Autodesk Inventor part; units mm, degrees
ref_plane "YZ Plane" through (0, 0, 0) normal (1, 0, 0) x (0, 1, 0)
ref_plane "XZ Plane" through (0, 0, 0) normal (0, 1, 0) x (-1, 0, 0)
ref_plane "XY Plane" through (0, 0, 0) normal (0, 0, 1) x (1, 0, 0)
sketch "Sketch1" plane through (0, 0, 0) normal (0, 1, 0) x (-1, 0, 0)
  circle A0 centre (0, 0) radius 45 construction
  line L0 (36.9, 6.3) -> (13, 6.3)
  line L1 (13, 6.3) -> (13, -6.3)
  line L2 (13, -6.3) -> (36.9, -6.3)
  line L3 (36.9, -6.3) -> (36.9, 6.3)
  line L4 (-12.994, 35.1063) -> (-23.906, 28.8063)
  line L5 (-23.906, 28.8063) -> (-11.956, 8.1083)
  line L6 (-1.044, 14.4083) -> (-12.994, 35.1063)
  line L7 (-11.956, 8.1083) -> (-1.044, 14.4083)
  line L8 (-18.9106, -20.1539) -> (-7.9987, -26.4539)
  line L9 (-7.9987, -26.4539) -> (3.9513, -5.7559)
  line L10 (-6.9606, 0.5441) -> (-18.9106, -20.1539)
  line L11 (3.9513, -5.7559) -> (-6.9606, 0.5441)
  circle A1 centre (11.0177, 0) radius 18 construction
  circle A2 centre (-5.5088, 9.5416) radius 18 construction
  circle A3 centre (-5.5088, -9.5416) radius 18 construction
  circle A4 centre (17, -29.4449) radius 1.8
  line L12 (0, 0) -> (20.2687, -35.1063)
  circle A5 centre (17, 29.4449) radius 1.8
  circle A6 centre (-34, 0) radius 1.8
  circle A7 centre (0, 0) radius 49
  line L13 (-5.5088, -9.5416) -> (-0.5088, -0.8813) construction
  line L14 (-5.5088, -9.5416) -> (4.4912, -9.5416) construction
  line L15 (-18.45, -31.9563) -> (3.4912, 6.0469) construction
  line L16 (-17.931, -18.4573) -> (-7.019, -24.7573) construction
  point P0 (-12.475, -21.6073)
  point P1 (-7.4794, -12.9547)
  dimension "d0" = 90
  dimension "d1" = 12.6
  dimension "d2" = 23.9
  dimension "d3" = 13
  dimension "d4" = 38.7
  dimension "d7" = 360
  dimension "d9" = 36
  dimension "d12" = 360
  dimension "d14" = 3.6
  dimension "d15" = 34
  dimension "d16" = -0.544
  dimension "d19" = 360
  dimension "d21" = 98
  dimension "d38" = 10
  dimension "d39" = 60
  dimension "d40" = 14.9588
extrude "Extrusion1" add sketch "Sketch1" along normal blind 7
sketch "Sketch2" plane through (0, 7, 0) normal (0, 1, 0) x (1, 0, 0)
  circle A0 centre (0, 0) radius 39.9 construction
  line L0 (1.044, -14.4083) -> (11.956, -8.1083) construction
  line L1 (6.5, -11.2583) -> (23.7787, -41.1859) construction
  circle A1 centre (19.95, -34.5544) radius 0.8
  circle A2 centre (14.95, 25.8942) radius 0.8
  circle A3 centre (-39.9, 0) radius 0.8
  line L2 (12.994, -35.1063) -> (1.044, -14.4083) construction
  line L3 (7.019, -24.7573) -> (17.931, -18.4573) construction
  line L4 (11.956, -8.1083) -> (23.906, -28.8063) construction
  circle A4 centre (5, -8.6603) radius 0.8
  circle A5 centre (0, 0) radius 0.8
  circle A6 centre (-10, 0) radius 0.8
  line L5 (0, 0) -> (22.1905, 38.4351) construction
  line L6 (0, 0) -> (44.3811, 0) construction
  line L7 (15.8257, 27.411) -> (10.8257, 18.7507)
  dimension "d24" = 79.8
  dimension "d25" = 1.6
  dimension "d28" = 360
  dimension "d34" = 360
  dimension "d41" = 60
  dimension "d42" = 10
extrude "Extrusion2" cut sketch "Sketch2" against normal through all
sketch "Sketch6" plane through (0, 7, 0) normal (0, 1, 0) x (1, 0, 0)
  line L0 (39.1506, 17.8109) -> (-4.1506, 42.8109)
  line L1 (-4.1506, 42.8109) -> (-39.1506, -17.8109)
  line L2 (-39.1506, -17.8109) -> (4.1506, -42.8109)
  line L3 (4.1506, -42.8109) -> (39.1506, 17.8109)
  line L4 (21.6506, -12.5) -> (-21.6506, 12.5) construction
  circle A0 centre (0, 0) radius 0.8 construction
  line L5 (0, 0) -> (-28.8675, 0) construction
  circle A1 centre (-39.1506, -17.8109) radius 1.8
  circle A2 centre (4.1506, -42.8109) radius 1.8
  circle A3 centre (-4.1506, 42.8109) radius 1.8
  circle A4 centre (39.1506, 17.8109) radius 1.8
  point P0 (0, 0)
  dimension "d43" = 25
  dimension "d44" = 25
  dimension "d45" = 35
  dimension "d46" = 35
  dimension "d47" = 30
  dimension "d48" = 3.6
  dimension "d49" = 3.6
extrude "Extrusion3" cut sketch "Sketch6" against normal through all contours L3 A4 L0 | L0 A4 L3 | A3 L1 L0 | L0 L1 A3 | A2 L2 L3 | L3 L2 A2 | A1 L2 L1 | L1 L2 A1
sketch "Sketch7" plane through (0, 7, 0) normal (0, 1, 0) x (1, 0, 0)
  circle A0 centre (-4.1506, 42.8109) radius 1.8
  circle A1 centre (-4.1506, 42.8109) radius 3.75
  circle A2 centre (39.1506, 17.8109) radius 1.8
  circle A3 centre (39.1506, 17.8109) radius 3.75
  circle A4 centre (-39.1506, -17.8109) radius 1.8
  circle A5 centre (-39.1506, -17.8109) radius 3.75
  circle A6 centre (4.1506, -42.8109) radius 1.8
  circle A7 centre (4.1506, -42.8109) radius 3.75
  point P0 (0, 0)
  dimension "d52" = 7.5
  dimension "d53" = 7.5
  dimension "d54" = 7.5
  dimension "d55" = 7.5
extrude "Extrusion4" cut sketch "Sketch7" against normal blind 2 contours A0 | A1 | A2 | A3 | A5 | A6 | A7
properties part number "Servo Mounts"
Design review of the part built by this model. Coordinates are the model's own, in mm. A direction names the side the tool comes from. Round coordinates to 2 decimals unless told otherwise and drop trailing zeros. Write each loop counter-clockwise with the first axis right and the second up, starting at its lowest first coordinate (ties: lowest second). Pieces come first, ordered by that corner, then holes.
Item 1: For faces 1 (the cylindrical face through (1.387, 6.014, 40.276)), 2 (the flat face through (1, 7, 1)), 3 (the flat face through (6.6, 3.5, 11.2)), list the 3-axis set-ups (+Z, -Z, +X, -X, +Y, -Y) from which the entire face can be reached by the end or side of a thin tool; tool diameter is ignored.
Item 2: Consider section A-A on x = 34. Give the boundary of the cut face in (y, z).
Item 3: For pin 1 Ø2 at (y, z) = (2, -2) entering from +X; pin 2 Ø1.5 at (x, y) = (8.5, 1) entering from -Z; pin 3 Ø4.5 at (x, z) = (39.15, -17.81) entering from +Y, all flat-tipped, find the tip position at first contact; note any pin that passes through.
Item 4: Consider section B-B on y = 3. Count the separate pieces of the cut face and the enclosed holes in it, and give its area (3 significant figures).
Item 5: Wall thickness on L1, parallel to Z at x = -40, y = 1.5; L2, parallel to Z at x = 0, y = 4.25; L3, parallel to X at y = 5.75, z = 16: over which ranges is each line inside the solid? List them lowest first.
Item 6: Consider section C-C on z = -34. Give the boundary of the cut face in (x, y).
Item 7: Draft analysis for pull direction X (two halves, no side actions). For faces 4 (the flat face through (18.015, 3.451, 18.602)), 5 (the cylindrical face through (-26.34, 3.45, -41.32)), 6 (the flat face through (1, 0, 1)), state which applies: released by +X, released by -X, zero draft, split by the parting line, or undercut.
Check values:
1. face 1: +Y
1. face 2: +Z, -Z, +X, -X, +Y
1. face 3: +Y, -Y
2. outline: (0, -35.28) - (7, -35.28) - (7, -1.8) - (0, -1.8) - close; (0, 1.8) - (7, 1.8) - (7, 35.28) - (0, 35.28) - close
3. pin 1: stops at x = 48.99
3. pin 2: stops at z = -48.38
3. pin 3: stops at y = 5
4. separate pieces: 1
4. enclosed holes: 16
4. area: 6,560 mm2
5. L1: z = -28.3 to -0.79, 0.79 to 16.22, 19.4 to 28.3
5. L2: z = -49 to -12.6, -3.47 to -0.8, 0.8 to 49
5. L3: x = -46.31 to -42.43, -35.87 to 1.96, 16.51 to 46.31
6. outline: (-35.28, 0) - (35.28, 0) - (35.28, 7) - (-35.28, 7) - close
7. face 4: undercut
7. face 5: split by the parting line
7. face 6: zero draft
